Geometry: see drawing. Coordinates: mm, zero at the bounding-box minimum. A direction names the side the tool comes from. Give positions to 0.01 mm unless a question says otherwise; leave off trailing zeros. Write each loop counter-clockwise with the first axis right and the second up, starting at its lowest first coordinate (ties: lowest second). Pieces come first, ordered by that corner, then holes. Notation, with made-up numbers: (69.5, 1.25) - (100.5, 1.25) arc R13 cw to (100.5, 9.25) - close; hole circle Ø11 at (13, -6.75). An arc over 180 degrees is marked (long way). Use a Markdown table: item, result. Add a question column.
1. Set-up query: the marked faces 1 and 2. Return all of +Z, -Z, +X, -X, +Y, -Y with unobstructed straight access to the full face (end or side cutting, diameter ignored); none if empty.
2. Material intervals for probe 1 along Z at (x, y) = (17.5, 17.25); probe 2 along X at (y, z) = (12, 17); probe 3 along Y at (x, z) = (20, 50), sorted ascending.
3. Section query D-D, the plane y = 23.5. Return loops of the section in (x, z), plus the area to 3 significant figures.
4. Section query A-A, the plane x = 12. Return loops of the section in (y, z) (3 decimals), plus the area to 3 significant figures.
5. Pin query (flat end, axial travel): pin 1 (12 mm diameter, centred on x = 6, z = 21, fed in from +Y); pin 2 (1.5 mm diameter, centred on y = 19, z = 36.5, fed in from +X); pin 3 (1 mm diameter, centred on x = 5, y = 9.5, fed in from +Z). Return the tip coordinate at first contact, or that it passes through.
6. Section query B-B, the plane y = 20.75. Return loops of the section in (x, z).
7. Section query C-C, the plane z = 5. Return loops of the section in (x, y) (3 decimals).
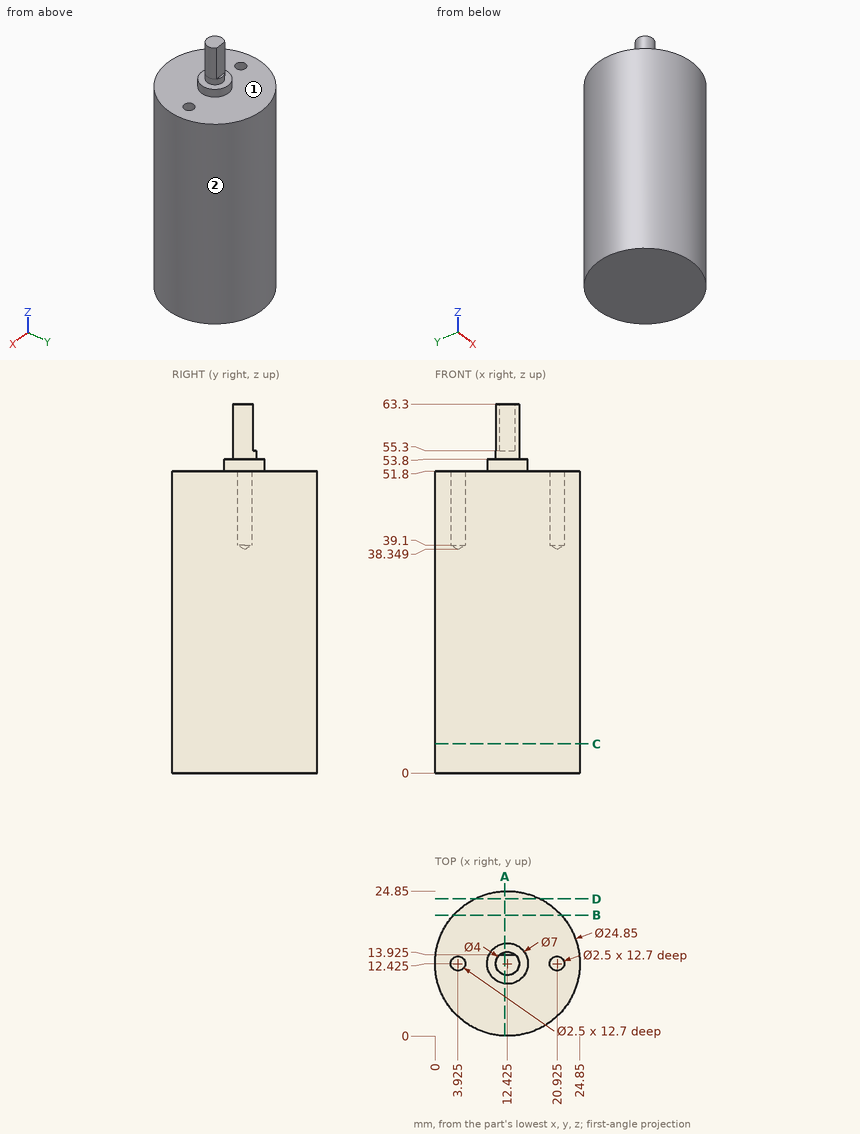
Result sheet:
| question | item | result |
|---|---|---|
| 1 | face 1 | +Z |
| 1 | face 2 | +Z, -Z |
| 2 | probe 1 | z = 0 to 51.8 |
| 2 | probe 2 | x = 0.01 to 24.84 |
| 2 | probe 3 | y = 2.58 to 11.58, 13.27 to 22.27 |
| 3 | outline | (6.79, 0) - (18.06, 0) - (18.06, 51.8) - (6.79, 51.8) - close |
| 3 | area | 584 mm² |
| 4 | outline | (0.007, 0) - (24.843, 0) - (24.843, 51.8) - (15.899, 51.8) - (15.899, 53.8) - (14.379, 53.8) - (14.379, 55.3) - (13.925, 55.3) - (13.925, 63.3) - (10.471, 63.3) - (10.471, 53.8) - (8.951, 53.8) - (8.951, 51.8) - (0.007, 51.8) - close |
| 4 | area | 1,330 mm² |
| 5 | pin 1 | stops at y = 24.84 |
| 5 | pin 2 | stops at x = 23.4 |
| 5 | pin 3 | stops at z = 51.8 |
| 6 | outline | (3.2, 0) - (21.65, 0) - (21.65, 51.8) - (3.2, 51.8) - close |
| 7 | outline | circle Ø24.85 at (12.425, 12.425) |
